Geometry: final body of the model. Coordinates: model frame, mm. A direction names the side the tool comes from. Give positions to 0.01 mm unless a question says otherwise; leave off trailing zeros. Write each loop counter-clockwise with the first axis right and the second up, starting at its lowest first coordinate (ties: lowest second). Pieces come first, ordered by that corner, then holes.
Q1. Section C-C (x = -17). Return the cut outline in (y, z), plus the area to 3 significant figures.
Q2. Pin query (flat end, axial travel): pin 1 Ø3.5 at (x, y) = (-31.85, 15.5) entering from -Z; pin 2 Ø1.2 at (y, z) = (-70, 0.5) entering from +X; pin 3 Ø1 at (x, y) = (8, -32) entering from +Z; pin 4 Ø2.5 at (x, y) = (-31.85, 15.5) entering from +Z. Return the tip coordinate at first contact, or that it passes through.
Q3. Section A-A (y = 6). Return the cut outline in (x, z).
Q4. Section B-B (z = -4). Return the cut outline in (x, y).
Q5. Reachability of faces 4 (the flat face through (37, -36.5, -8)), 5 (the cylindrical face through (-32.5, 18.43, -9.72)), 6 (the flat face through (-35.4, 15, 0)) from +Z, -Z, +X, -X, +Y, -Y: full face, straight path, thin tool, end or side. Return the list, or none.
Q6. Line query: line 1 (X direction, y = -20, z = -3.75); line 2 (Y direction, x = -31, z = -10); line 3 (Y direction, x = 23, z = -7). Output: solid intervals per line, ascending.
Q7. Mould query, pull axis X, two halves, no side actions, for faces 1 (the flat face through (-30, -72, 1.6)), 2 (the cylindrical face through (35.294, -76.219, -5.451)), 3 (the cylindrical face through (34.62, -71.35, -9.72)). Classes: +X half, -X half, draft (parallel to the pull), parting line (faces both ways), or undercut.
Q8. Section D-D (y = -34). Return the cut outline in (x, z).
from build123d import *

# Parameters (mm, degrees)
PAD014_DEPTH    = 9
FILLET012_R     = 2
SKETCH024_R     = 3
POCKET009_DEPTH = 2.6
SKETCH025_R     = 1.6
POCKET010_DEPTH = 7
SKETCH026_R     = 1.6
PAD015_DEPTH    = 3.6
SKETCH027_W     = 2
SKETCH027_H     = 21
SKETCH027_W_2   = 7
SKETCH027_H_2   = 2
PAD016_DEPTH    = 5.4
SKETCH028_W     = 20
SKETCH028_H     = 2
POCKET011_DEPTH = 77.701


with BuildPart() as part:
    # Sketch023 → Pad014 (new body)
    with BuildSketch(Plane.XY):
        with BuildLine():
            Line((-33.7, 21.5), (33.7, 21.5))
            ThreePointArc((37.7, 17.5), (36.528427, 20.328427), (33.7, 21.5))
            Line((37.7, 17.5), (37.7, -70.5))
            ThreePointArc((29.7, -78.5), (35.356854, -76.156854), (37.7, -70.5))
            Line((29.7, -78.5), (-29.7, -78.5))
            ThreePointArc((-37.7, -70.5), (-35.356854, -76.156854), (-29.7, -78.5))
            Line((-37.7, -70.5), (-37.7, 17.5))
            ThreePointArc((-33.7, 21.5), (-36.528427, 20.328427), (-37.7, 17.5))
        make_face()
    extrude(amount=-PAD014_DEPTH)

    # Fillet012
    fillet012_edges = [part.edges().sort_by_distance(p)[0] for p in [
        (0, 21.5, -9),
    ]]
    fillet(fillet012_edges, radius=FILLET012_R)

    # Sketch024 (on Face8 of Fillet012) → Pocket009 (cut)
    with BuildSketch(Plane(origin=(0, 0, -9), x_dir=(1, 0, 0), z_dir=(0, 0, -1))):
        with Locations((-31.85, 72.5)):
            Circle(SKETCH024_R)
        with Locations((31.85, 72.5)):
            Circle(SKETCH024_R)
        with Locations((-31.85, -15.5)):
            Circle(SKETCH024_R)
        with Locations((31.85, -15.5)):
            Circle(SKETCH024_R)
    extrude(amount=-POCKET009_DEPTH, mode=Mode.SUBTRACT)

    # Sketch025 (on Face4 of Pocket009) → Pocket010 (cut)
    with BuildSketch(Plane.XY):
        with Locations((-31.85, 15.5)):
            Circle(SKETCH025_R)
        with Locations((31.85, 15.5)):
            Circle(SKETCH025_R)
        with Locations((31.85, -72.5)):
            Circle(SKETCH025_R)
        with Locations((-31.85, -72.5)):
            Circle(SKETCH025_R)
        with BuildLine():
            Line((-31.85, 12.1), (-35.7, 12.1))
            Line((-35.7, 12.1), (-35.7, -69.1))
            Line((-35.7, -69.1), (-31.85, -69.1))
            ThreePointArc((-28.45, -72.5), (-29.445837, -70.095837), (-31.85, -69.1))
            Line((-28.45, -76.5), (-28.45, -72.5))
            Line((-28.45, -76.5), (28.45, -76.5))
            Line((28.45, -76.5), (28.45, -72.5))
            ThreePointArc((31.85, -69.1), (29.445837, -70.095837), (28.45, -72.5))
            Line((35.7, -69.1), (31.85, -69.1))
            Line((35.7, -69.1), (35.7, 12.1))
            Line((35.7, 12.1), (31.85, 12.1))
            ThreePointArc((28.45, 15.5), (29.445837, 13.095837), (31.85, 12.1))
            Line((28.45, 19.5), (28.45, 15.5))
            Line((28.45, 19.5), (-28.45, 19.5))
            Line((-28.45, 19.5), (-28.45, 15.5))
            ThreePointArc((-31.85, 12.1), (-29.445837, 13.095837), (-28.45, 15.5))
        make_face()
    extrude(amount=-POCKET010_DEPTH, mode=Mode.SUBTRACT)

    # Sketch026 (on Face4 of Pocket010) → Pad015 (join)
    with BuildSketch(Plane.XY):
        with BuildLine():
            Line((-31.85, 12.1), (-35.4, 12.1))
            Line((-35.4, 12.1), (-35.4, 17.2))
            ThreePointArc((-33.4, 19.2), (-34.814214, 18.614214), (-35.4, 17.2))
            Line((-28.45, 19.2), (-33.4, 19.2))
            Line((-28.45, 19.2), (-28.45, 15.5))
            ThreePointArc((-31.85, 12.1), (-29.445837, 13.095837), (-28.45, 15.5))
        make_face()
        with Locations((-31.85, 15.5)):
            Circle(SKETCH026_R, mode=Mode.SUBTRACT)
        with BuildLine():
            Line((35.4, 12.1), (31.85, 12.1))
            ThreePointArc((28.45, 15.5), (29.445837, 13.095837), (31.85, 12.1))
            Line((28.45, 19.2), (28.45, 15.5))
            Line((28.45, 19.2), (33.4, 19.2))
            ThreePointArc((35.4, 17.2), (34.814214, 18.614214), (33.4, 19.2))
            Line((35.4, 12.1), (35.4, 17.2))
        make_face()
        with Locations((31.85, 15.5)):
            Circle(SKETCH026_R, mode=Mode.SUBTRACT)
        with BuildLine():
            Line((28.45, -76.2), (28.45, -72.5))
            ThreePointArc((31.85, -69.1), (29.445837, -70.095837), (28.45, -72.5))
            Line((35.4, -69.1), (31.85, -69.1))
            Line((35.4, -69.1), (35.4, -70.2))
            ThreePointArc((29.4, -76.2), (33.642641, -74.442641), (35.4, -70.2))
            Line((28.45, -76.2), (29.4, -76.2))
        make_face()
        with Locations((31.85, -72.5)):
            Circle(SKETCH026_R, mode=Mode.SUBTRACT)
        with BuildLine():
            Line((-35.4, -69.1), (-31.85, -69.1))
            ThreePointArc((-28.45, -72.5), (-29.445837, -70.095837), (-31.85, -69.1))
            Line((-28.45, -76.2), (-28.45, -72.5))
            Line((-28.45, -76.2), (-29.4, -76.2))
            ThreePointArc((-35.4, -70.2), (-33.642641, -74.442641), (-29.4, -76.2))
            Line((-35.4, -69.1), (-35.4, -70.2))
        make_face()
        with Locations((-31.85, -72.5)):
            Circle(SKETCH026_R, mode=Mode.SUBTRACT)
    extrude(amount=PAD015_DEPTH)

    # Sketch027 (on Face4 of Pad015) → Pad016 (join)
    with BuildSketch(Plane.XY):
        with Locations((-36.7, 0)):
            Rectangle(SKETCH027_W, SKETCH027_H)
        with Locations((36.7, 0)):
            Rectangle(SKETCH027_W, SKETCH027_H)
        with Locations((-22, 20.5)):
            Rectangle(SKETCH027_W_2, SKETCH027_H_2)
    extrude(amount=PAD016_DEPTH)

    # Sketch028 → Pocket011 (cut, through all)
    with BuildSketch(Plane.YZ.offset(40)):
        with Locations((-46.5, -5.8)):
            Rectangle(SKETCH028_W, SKETCH028_H)
        with Locations((1.5, -5.8)):
            Rectangle(SKETCH028_W, SKETCH028_H)
    extrude(amount=-POCKET011_DEPTH, mode=Mode.SUBTRACT)


with BuildPart() as part_1:
    # Body006 placement: moved
    add(part.part.moved(Location((0, 0, -2))))


solid = part_1.part
Computed:
1. outline: (-78.5, -9) arc R2 ccw to (-76.5, -11) - (19.5, -11) arc R2 ccw to (21.5, -9) - (21.5, -2) - (19.5, -2) - (19.5, -9) - (-76.5, -9) - (-76.5, -2) - (-78.5, -2) - close
1. area: 226 mm2
2. pin 1: stops at z = -8.4
2. pin 2: stops at x = 35.4
2. pin 3: stops at z = -9
2. pin 4: passes through
3. outline: (-37.7, -9) arc R2 ccw to (-35.7, -11) - (35.7, -11) arc R2 ccw to (37.7, -9) - (37.7, -8.8) - (35.7, -8.8) - (35.7, -9) - (-35.7, -9) - (-35.7, -8.8) - (-37.7, -8.8) - close; (-37.7, -6.8) - (-35.7, -6.8) - (-35.7, 3.4) - (-37.7, 3.4) - close; (35.7, -6.8) - (37.7, -6.8) - (37.7, 3.4) - (35.7, 3.4) - close
4. outline: (-37.7, -70.5) arc R8 ccw to (-29.7, -78.5) - (29.7, -78.5) arc R8 ccw to (37.7, -70.5) - (37.7, 17.5) arc R4 ccw to (33.7, 21.5) - (-33.7, 21.5) arc R4 ccw to (-37.7, 17.5) - close; hole (-35.7, -69.1) - (-31.85, -69.1) arc R3.4 cw to (-28.45, -72.5) - (-28.45, -76.5) - (28.45, -76.5) - (28.45, -72.5) arc R3.4 cw to (31.85, -69.1) - (35.7, -69.1) - (35.7, 12.1) - (31.85, 12.1) arc R3.4 cw to (28.45, 15.5) - (28.45, 19.5) - (-28.45, 19.5) - (-28.45, 15.5) arc R3.4 cw to (-31.85, 12.1) - (-35.7, 12.1) - close; hole circle Ø3.2 at (-31.85, -72.5); hole circle Ø3.2 at (-31.85, 15.5); hole circle Ø3.2 at (31.85, -72.5); hole circle Ø3.2 at (31.85, 15.5)
5. face 4: +X, -X
5. face 5: -Z
5. face 6: +Z, -X, +Y, -Y
6. line 1: x = -37.7 to -35.7, 35.7 to 37.7
6. line 2: y = -78.12 to -75.38, -69.62 to 12.62, 18.38 to 21.23
6. line 3: y = -78.5 to -76.5, 19.5 to 21.5
7. face 1: draft
7. face 2: +X half
7. face 3: undercut
8. outline: (-37.7, -9) arc R2 ccw to (-35.7, -11) - (35.7, -11) arc R2 ccw to (37.7, -9) - (37.7, -2) - (35.7, -2) - (35.7, -9) - (-35.7, -9) - (-35.7, -2) - (-37.7, -2) - close
